Can you work these out from the model? Positions are in its coordinate system, mm. Round coordinates to 2 decimals unless told otherwise and drop trailing zeros. Order: outer loops, then holes, each group sorted by start corner. A loop starts at its lowest first (then second) coordinate and runs counter-clockwise, first axis right, second up. Notation, with made-up numbers: (84, 0) -> (135, 0) arc R12 ccw to (135, 4) -> close; hole circle Ø4 at (-20.75, -4.5). An arc over 180 degrees is marked (long way). One line per item, written item: value.
Autodesk Inventor part; units mm, degrees
sketch "Эскиз1" plane through (0, 0, 0) normal (0, 0, 1) x (1, 0, 0)
  line L0 (0, 613.0143) -> (0, -102.169)
  line L1 (-210, 0) -> (1260, 0)
  line L2 (0, 0) -> (50, 0)
  line L3 (1050, 510.8452) -> (0, 510.8452)
  line L4 (0, 0) -> (0, 510.8452)
  line L5 (1050, 510.8452) -> (1050, 267.9492)
  line L6 (1050, 267.9492) -> (50, 0)
  dimension "d7" = 1050
  dimension "d8" = 50
  dimension "d9" = 15
extrude "Выдавливание1" add sketch "Эскиз1" along normal mid plane 10
properties part number "ДетальДударь"
Q1. I want a section at A-A on z = -0.75. List the corners of the cut face in (x, y) for me, plus the area to 3 significant figures.
Answers below:
outline: (0, 0) -> (50, 0) -> (1050, 267.95) -> (1050, 510.85) -> (0, 510.85) -> close
area: 402,000 mm^2
Q2. Please list where these lines run through material, in increasing order: line 1 along Y through (x, z) = (383.5, 2); line 2 along Y through (x, z) = (832, -0.75).
Answers below:
line 1: 89.36 to 510.85
line 2: 209.54 to 510.85
Q3. Will this pin go through, and if not, where does the flat tip stop? pin 1 Ø3 at (y, z) = (101.5, 3) entering from -X.
Answers below:
pin 1: x = 0
Q4. I want a section at B-B on x = 604. List the corners of the cut face in (y, z) for me.
Answers below:
outline: (148.44, -5) -> (510.85, -5) -> (510.85, 5) -> (148.44, 5) -> close
Q5. I want a section at C-C on y = 43. List the corners of the cut face in (x, z) for me, plus the area to 3 significant figures.
Answers below:
outline: (0, -5) -> (210.48, -5) -> (210.48, 5) -> (0, 5) -> close
area: 2,100 mm^2
